```python
from build123d import *

# Parameters (mm, degrees)
F1_DEPTH = 742.95
F2_R     = 1.5875
F3_R     = 0.635


with BuildPart() as f1:
    # F0 (on Front) → F1 (new body, symmetric)
    with BuildSketch(Plane.XZ):
        with BuildLine():
            Line((0, 37.3126), (0, 0))
            Line((0, 0), (41.275, 0))
            Line((41.275, 0), (41.275, 37.3126))
            ThreePointArc((41.275, 37.3126), (37.3126, 41.275), (33.3502, 37.3126))
            Line((33.3502, 37.3126), (34.9377, 37.3126))
            ThreePointArc((34.9377, 37.3126), (37.3126, 39.6875), (39.6875, 37.3126))
            Line((39.6875, 37.3126), (39.6875, 1.5875))
            Line((39.6875, 1.5875), (1.5875, 1.5875))
            Line((1.5875, 1.5875), (1.5875, 37.3126))
            ThreePointArc((1.5875, 37.3126), (3.9624, 39.6875), (6.3373, 37.3126))
            Line((6.3373, 37.3126), (7.9248, 37.3126))
            ThreePointArc((7.9248, 37.3126), (3.9624, 41.275), (0, 37.3126))
        make_face()
    extrude(amount=F1_DEPTH, both=True)

    # F2
    f2_edges = [f1.edges().sort_by_distance(p)[0] for p in [
        (1.5875, 0, 1.5875),
        (39.6875, 0, 1.5875),
        (0, 0, 0),
        (41.275, 0, 0),
    ]]
    fillet(f2_edges, radius=F2_R)

    # F3
    f3_edges = [f1.edges().sort_by_distance(p)[0] for p in [
        (7.13105, 742.95, 37.3126),
        (7.9248, 0, 37.3126),
        (7.13105, -742.95, 37.3126),
        (6.3373, 0, 37.3126),
        (33.3502, 0, 37.3126),
        (34.9377, 0, 37.3126),
    ]]
    fillet(f3_edges, radius=F3_R)


solid = f1.part
```
Source: CAD feature listing. Evaluate the final solid. Frame: model axes, mm. A direction names the side the tool comes from. Give positions to 0.01 mm unless a question says otherwise; leave off trailing zeros. Loops run counter-clockwise (first coordinate to the right, second up) from the corner with the lowest first, then second, coordinate; pieces in that order, holes last. Notation, with made-up numbers: (75.5, -31.75) -> (88.5, -31.75) arc R21 cw to (88.5, -24.75) -> close; hole circle Ø3 at (4.25, 38). An arc over 180 degrees is marked (long way). Use a Markdown table: item, result. Add a question column.
(1) First-contact query: pin 1 Ø4 at (x, z) = (37, 14) entering from -Y; pin 2 Ø1.5 at (x, y) = (29, 244.5) entering from +Z. Flat tips, straight axial feed; report the tip coordinate or a pass-through.
(2) Access query for faces 4 (the face through (39.688, -10, 20)), 5 (the face through (21, 742.95, 1)). Directions: +Z, -Z, +X, -X, +Y, -Y. A direction counts if a zero-diameter tool reaches every point of the face in a straight line with its end or side. Return the directions, or none.
(3) Section query C-C (x = 25.5). Output: boundary loops of the cut face in (y, z), then the cut area to 3 significant figures.
(4) Ray query, line 1 (X direction, y = 428, z = 37.5); line 2 (X direction, y = 428.5, z = 29) (1 decimal); line 3 (Z direction, x = 34, y = -351). Return the intervals inside material, ascending.
(5) Pull-direction query (X, two-part tool) for faces 1 (the face through (1.588, -10, 20)), 2 (the face through (0, -10, 20)), 3 (the face through (20, -10, 0)); classes: +X half, -X half, draft (parallel to the pull), parting line (faces both ways), or undercut.
Checked values:
| question | item | result |
|---|---|---|
| 1 | pin 1 | through |
| 1 | pin 2 | z = 1.59 |
| 2 | face 4 | +Y, -Y |
| 2 | face 5 | +Z, -Z, +X, -X, +Y |
| 3 | outline | (-742.95, 0) -> (742.95, 0) -> (742.95, 1.59) -> (-742.95, 1.59) -> close |
| 3 | area | 2,360 mm^2 |
| 4 | line 1 | 0 to 1.59, 6.45 to 7.68, 33.6 to 34.82, 39.68 to 41.27 |
| 4 | line 2 | 0 to 1.6, 39.7 to 41.3 |
| 4 | line 3 | 0 to 1.59, 37.31 to 39.49 |
| 5 | face 1 | undercut |
| 5 | face 2 | -X half |
| 5 | face 3 | draft |
